from build123d import *

# Parameters (mm, degrees)
SKETCH1_W           = 99.8
SKETCH1_H           = 40
SKETCH1_W_2         = 10
SKETCH1_H_2         = 3
BOSS_EXTRUDE1_DEPTH = 3
SKETCH2_R           = 1.1
CUT_EXTRUDE1_DEPTH  = 76.977118266
SKETCH3_W           = 40
SKETCH3_H           = 20
CUT_EXTRUDE2_DEPTH  = 76.977118266
FILLET1_R           = 2


with BuildPart() as part:
    # Sketch1 → Boss-Extrude1 (new body)
    with BuildSketch(Plane(origin=(0, 0, 0), x_dir=(0, 0, -1), z_dir=(1, 0, 0))):
        with Locations((22.45, 0)):
            Rectangle(SKETCH1_W, SKETCH1_H)
        with Locations((-22.45, 21.5)):
            Rectangle(SKETCH1_W_2, SKETCH1_H_2)
        with Locations((22.45, 21.5)):
            Rectangle(SKETCH1_W_2, SKETCH1_H_2)
        with Locations((67.35, 21.5)):
            Rectangle(SKETCH1_W_2, SKETCH1_H_2)
        with Locations((67.35, -21.5)):
            Rectangle(SKETCH1_W_2, SKETCH1_H_2)
        with Locations((22.45, -21.5)):
            Rectangle(SKETCH1_W_2, SKETCH1_H_2)
        with Locations((-22.45, -21.5)):
            Rectangle(SKETCH1_W_2, SKETCH1_H_2)
    extrude(amount=BOSS_EXTRUDE1_DEPTH)

    # Sketch2 → Cut-Extrude1 (cut, through all)
    with BuildSketch(Plane(origin=(3, 0, 0), x_dir=(0, 0, -1), z_dir=(1, 0, 0))):
        with Locations((-20.5, 8)):
            Circle(SKETCH2_R)
        with Locations((-20.5, -8)):
            Circle(SKETCH2_R)
        with Locations((20.5, 8)):
            Circle(SKETCH2_R)
        with Locations((20.5, -8)):
            Circle(SKETCH2_R)
        with BuildLine():
            Line((-13, 8.1), (13, 8.1))
            ThreePointArc((13, 8.1), (21.1, 0), (13, -8.1))
            Line((13, -8.1), (-13, -8.1))
            ThreePointArc((-13, -8.1), (-21.1, 0), (-13, 8.1))
        make_face()
    extrude(amount=-CUT_EXTRUDE1_DEPTH, mode=Mode.SUBTRACT)

    # Sketch3 → Cut-Extrude2 (cut, through all)
    with BuildSketch(Plane(origin=(3, 0, 0), x_dir=(0, 0, -1), z_dir=(1, 0, 0))):
        with Locations((43.5, -7)):
            Rectangle(SKETCH3_W, SKETCH3_H)
    extrude(amount=-CUT_EXTRUDE2_DEPTH, mode=Mode.SUBTRACT)

    # Fillet1
    fillet1_edges = [part.edges().sort_by_distance(p)[0] for p in [
        (1.5, -17, -23.5),
        (1.5, 3, -23.5),
        (1.5, 3, -63.5),
        (1.5, -17, -63.5),
    ]]
    fillet(fillet1_edges, radius=FILLET1_R)


solid = part.part
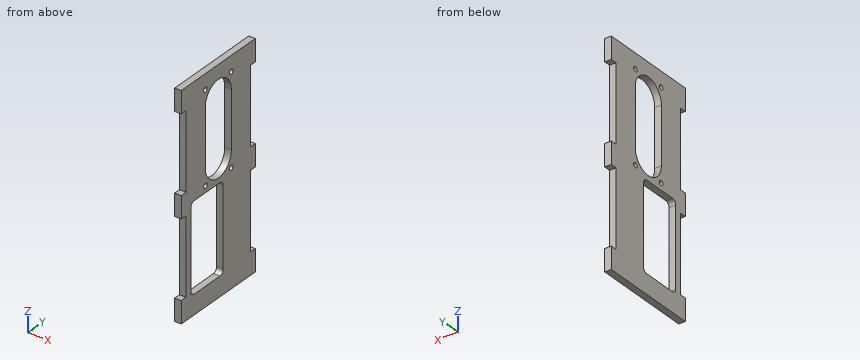
The listing builds one solid part. Answer for the finished solid, in the listing's coordinates (mm). Round coordinates to 2 decimals unless told otherwise and drop trailing zeros. Write each loop counter-clockwise with the first axis right and the second up, starting at its lowest first coordinate (ties: lowest second). Pieces come first, ordered by that corner, then holes. Notation, with made-up numbers: (3.25, 49.5) - (58.25, 49.5) arc R26 cw to (58.25, 67.5) - close; hole circle Ø9 at (58, 11.5). An arc over 180 degrees is marked (long way). Use a Markdown table: item, result. Add a question column.
1. The part is cut by section B-B (y = -13.5). Write down the section's boundary in (x, z), and give its area (3 significant figures).
2. The part is cut by section A-A (z = -39). Write down the section's boundary in (x, y).
3. Consider line 1 (Y direction, x = 0.95, z = -33.5); line 2 (Y direction, x = 0.65, z = 20.5); line 3 (Z direction, x = 1.9, y = -2.5). Determine where each line is inside the solid, lowest interval first.
4. Flat-ended cylindrical pins translate along their axes: P1, Ø1.5, axis at x = 1, z = -42.5, coming from the +Y side; P2, Ø1.8, axis at y = -8, z = -20.5, coming from the +X side; P3, Ø1.5, axis at x = 1, z = 5.5, coming from the -Y side; P4, Ø12, axis at y = 17, z = -40, coming from the -X side. Find the tip coordinate at first contact, or state that the pin passes through.
5. The part is cut by section C-C (x = 0.7). Give the number of separate pieces and of enclosed holes in the cut face, and give its area (3 significant figures).
Reported:
| question | item | result |
|---|---|---|
| 1 | outline | (0, -72.35) - (3, -72.35) - (3, -63.5) - (0, -63.5) - close; (0, -23.5) - (3, -23.5) - (3, 27.45) - (0, 27.45) - close |
| 1 | area | 179 mm^2 |
| 2 | outline | (0, -20) - (3, -20) - (3, -17) - (0, -17) - close; (0, 3) - (3, 3) - (3, 20) - (0, 20) - close |
| 3 | line 1 | -20 to -17, 3 to 20 |
| 3 | line 2 | -23 to -9.1, -6.9 to -3.06, 3.06 to 6.9, 9.1 to 23 |
| 3 | line 3 | -72.35 to -63.5, -23.5 to -20.7, 20.7 to 27.45 |
| 4 | P1 | y = 20 |
| 4 | P2 | through |
| 4 | P3 | y = -20 |
| 4 | P4 | x = 0 |
| 5 | separate pieces | 1 |
| 5 | enclosed holes | 6 |
| 5 | area | 2,730 mm^2 |
